The drawing under review shows one solid part. Ordinate dimensions are in mm from its lowest x, y, z. Give positions to 0.01 mm unless a question says otherwise; leave off trailing zeros. Write each loop counter-clockwise with the first axis right and the second up, starting at its lowest first coordinate (ties: lowest second). Pieces come first, ordered by that corner, then holes. Notation, with made-up numbers: M 47,31 L 91,31 A21 cw 91,45 Z; hole C 57.5,76.25 d11. An arc over 180 degrees is marked long. Answer as a JSON object with one key per item and string values. Group by question number.
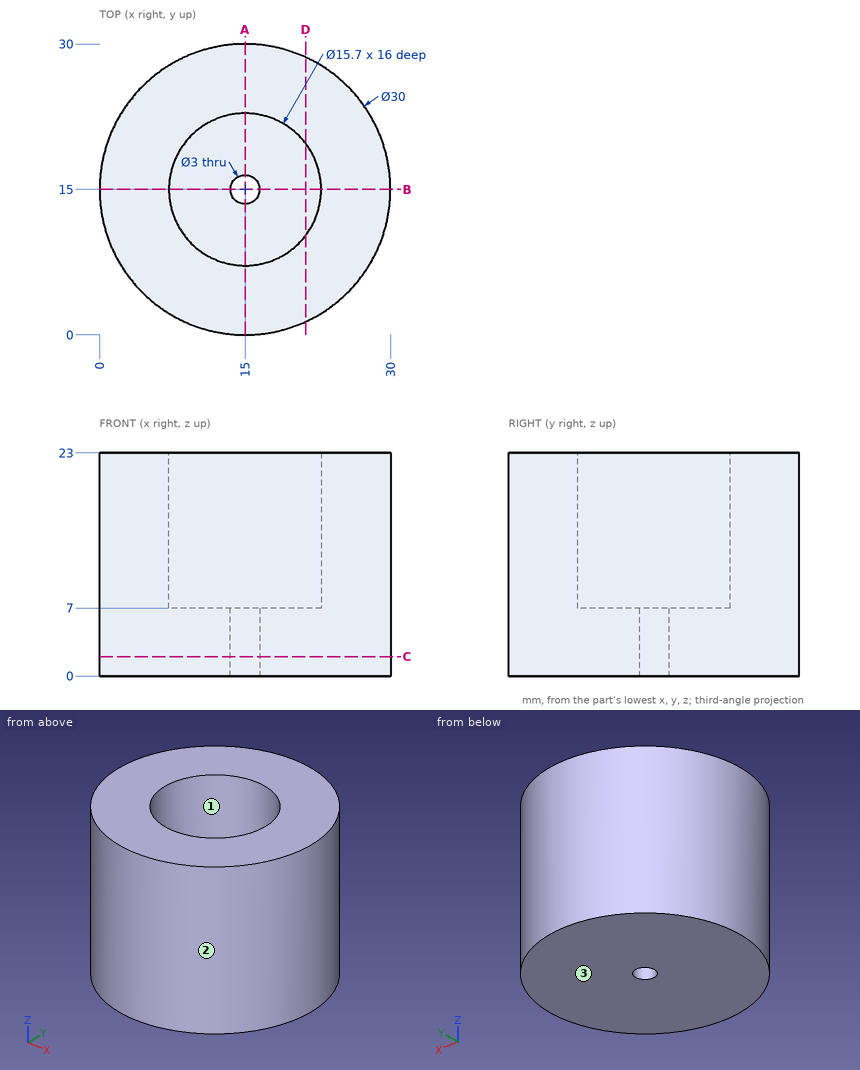
Item 1: Consider section C-C (z = 2). Give the boundary of the cut face in (x, y), plus the area to 3 significant figures.
Item 2: Consider section A-A (x = 15). Give the boundary of the cut face in (y, z), plus the area to 3 significant figures.
Item 3: Consider section D-D (x = 21.25). Give the boundary of the cut face in (y, z).
Item 4: To check wall thickness, follow probe 1 along Y at (x, z) = (15, 5.5); probe 2 along Y at (x, z) = (15, 17.75); probe 3 along X at (y, z) = (11, 11.5). State the ranges of each line that lie inside material, in increasing order.
Item 5: Insertion check: P1, Ø2, axis at y = 8, z = 9, coming from the -X side; P2, Ø1, axis at x = 24, z = 16, coming from the +Y side; P3, Ø1.5, axis at x = 21, y = 17, coming from the +Z side. Each pin has a flat end and moves straight along its axis. Give the tip position at first contact, or say it passes through.
Item 6: Draft analysis for pull direction Y (two halves, no side actions). For the marked faces 1, 2 and 3, state which applies: released by +Y, released by -Y, zero draft, split by the parting line, or undercut.
Result set:
{
 "1": {"outline": "C 15,15 d30; hole C 15,15 d3", "area": "700 mm^2"},
 "2": {"outline": "M 0,0 L 13.5,0 L 13.5,7 L 7.15,7 L 7.15,23 L 0,23 Z; M 16.5,0 L 30,0 L 30,23 L 22.85,23 L 22.85,7 L 16.5,7 Z", "area": "418 mm^2"},
 "3": {"outline": "M 1.36,0 L 28.64,0 L 28.64,23 L 19.75,23 L 19.75,7 L 10.25,7 L 10.25,23 L 1.36,23 Z"},
 "4": {"probe 1": "y = 0 to 13.5, 16.5 to 30", "probe 2": "y = 0 to 7.15, 22.85 to 30", "probe 3": "x = 0.54 to 8.25, 21.75 to 29.46"},
 "5": {"P1": "stops at x = 1.25", "P2": "stops at y = 27.36", "P3": "stops at z = 7"},
 "6": {"face 1": "undercut", "face 2": "split by the parting line", "face 3": "zero draft"}
}
